For this review, take the finished solid that the model builds, in its own axes (mm). Round coordinates to 2 decimals unless told otherwise and drop trailing zeros. Order: outer loops, then holes, each group sorted by start corner. A loop starts at its lowest first (then second) coordinate and runs counter-clockwise, first axis right, second up. Notation, with made-up numbers: (75.25, -22) -> (105.25, -22) arc R26 ccw to (105.25, 16) -> close; hole circle Ø11 at (-4, -30). An arc over 180 degrees is marked (long way). Put each result on its own line as item: value. Start each with the question number.
Autodesk Inventor part; units mm, degrees
ref_plane "YZ Plane" through (0, 0, 0) normal (1, 0, 0) x (0, 1, 0)
ref_plane "XZ Plane" through (0, 0, 0) normal (0, 1, 0) x (-1, 0, 0)
ref_plane "XY Plane" through (0, 0, 0) normal (0, 0, 1) x (1, 0, 0)
sketch "Sketch1" plane through (0, 0, 0) normal (0, 1, 0) x (-1, 0, 0)
  line L0 (0, 31.75) -> (162.56, 31.75)
  line L1 (162.56, 31.75) -> (162.56, -31.75)
  line L2 (162.56, -31.75) -> (0, -31.75)
  line L3 (0, -31.75) -> (0, 31.75)
  circle A0 centre (101.6, 0) radius 9.525
  point P0 (0, 0)
  point P1 (0, 0)
  dimension "d0" = 162.56
  dimension "d1" = 63.5
  dimension "d5" = 19.05
  dimension "d6" = 60.96
  dimension "d7" = 31.75
extrude "Extrusion1" add sketch "Sketch1" along normal blind 12.7
properties part number "Part3 x 2"
Item 1: For L1, parallel to Z at x = -101.6, y = 5 (3 decimals); L2, parallel to X at y = 1, z = -4; L3, parallel to Z at x = -109.5, y = 6.5, list the stretches that pass through material, from the lowest coordinate up.
Item 2: Mouldability with a two-part tool opening along Z and no side actions: class faces 1 (the face through (-80, 0, 0)), 2 (the face through (-92.084, 6.261, -0.419)), 3 (the face through (-80, 6, 31.75)) as +Z half, -Z half, draft (parallel to the pull), parting line (faces both ways), or undercut.
Item 3: Consider section B-B, the plane z = 0. Write out the cut boundary in (x, y) (3 decimals), plus the area to 3 significant figures.
Item 4: Consider section C-C, the plane y = 9.75. Write out the cut boundary in (x, z) (3 decimals), plus the area to 3 significant figures.
Item 5: Consider section A-A, the plane x = -101.6. Write out the cut boundary in (y, z) (3 decimals).
Evaluation:
1. L1: z = -31.75 to -9.525, 9.525 to 31.75
1. L2: x = -162.56 to -110.24, -92.96 to 0
1. L3: z = -31.75 to -5.32, 5.32 to 31.75
2. face 1: draft
2. face 2: undercut
2. face 3: +Z half
3. outline: (-162.56, 0) -> (-111.125, 0) -> (-111.125, 12.7) -> (-162.56, 12.7) -> close; (-92.075, 0) -> (0, 0) -> (0, 12.7) -> (-92.075, 12.7) -> close
3. area: 1,820 mm^2
4. outline: (-162.56, -31.75) -> (0, -31.75) -> (0, 31.75) -> (-162.56, 31.75) -> close; hole circle Ø19.05 at (-101.6, 0)
4. area: 10,000 mm^2
5. outline: (0, -31.75) -> (12.7, -31.75) -> (12.7, -9.525) -> (0, -9.525) -> close; (0, 9.525) -> (12.7, 9.525) -> (12.7, 31.75) -> (0, 31.75) -> close
